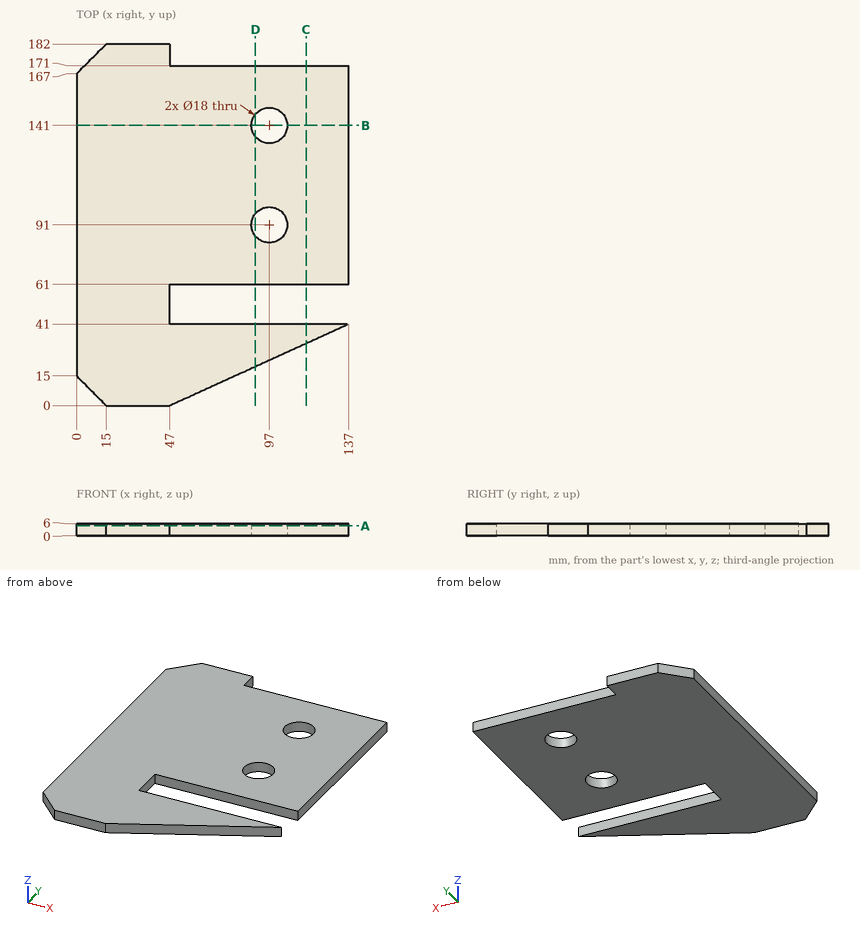
The figure shows three views and two pictorial views of one solid part (mm, origin at its lowest corner). Answer the questions. Round coordinates to 2 decimals unless told otherwise and drop trailing zeros. Write each loop counter-clockwise with the first axis right and the second up, starting at its lowest first coordinate (ties: lowest second). Pieces come first, ordered by that corner, then holes. Notation, with made-up numbers: (26, 64.25) - (51, 64.25) arc R11 ccw to (51, 72.25) - close; hole circle Ø5 at (17.5, 84.5). An arc over 180 degrees is marked (long way). Use one line per item in the form item = value. Start each with the question number.
Item 1: Find the intervals of material crossed by line 1 (X direction, y = 91, z = 2.55); line 2 (Y direction, x = 97, z = 4.05); line 3 (X direction, y = 57, z = 1.1), in increasing order. Write a range as [from, to].
Item 2: A cutting plane is placed at B-B (y = 141). Write down the section's boundary in (x, z), plus the area to 3 significant figures.
Item 3: Flat-ended cylindrical pins translate along their axes: pin 1 Ø3 at (y, z) = (47.5, 4) entering from +X; pin 2 Ø1.8 at (x, z) = (85, 3) entering from +Y; pin 3 Ø1.5 at (x, z) = (99.5, 1) entering from -Y (3 decimals). Find the tip coordinate at first contact, or state that the pin passes through.
Item 4: A cutting plane is placed at C-C (x = 115.5). Write down the section's boundary in (y, z).
Item 5: A cutting plane is placed at D-D (x = 90). Write down the section's boundary in (y, z), plus the area to 3 significant figures.
Item 6: A cutting plane is placed at A-A (z = 4.95). Write down the section's boundary in (x, y), plus the area to 3 significant figures.
The answers:
q1.line_1 = [0, 88], [106, 137]
q1.line_2 = [22.78, 41], [61, 82], [100, 132], [150, 171]
q1.line_3 = [0, 47]
q2.outline = (0, 0) - (88, 0) - (88, 6) - (0, 6) - close; (106, 0) - (137, 0) - (137, 6) - (106, 6) - close
q2.area = 714 mm^2
q3.pin_1 = 47
q3.pin_2 = 171
q3.pin_3 = 23.575
q4.outline = (31.21, 0) - (41, 0) - (41, 6) - (31.21, 6) - close; (61, 0) - (171, 0) - (171, 6) - (61, 6) - close
q5.outline = (19.59, 0) - (41, 0) - (41, 6) - (19.59, 6) - close; (61, 0) - (85.34, 0) - (85.34, 6) - (61, 6) - close; (96.66, 0) - (135.34, 0) - (135.34, 6) - (96.66, 6) - close; (146.66, 0) - (171, 0) - (171, 6) - (146.66, 6) - close
q5.area = 653 mm^2
q6.outline = (0, 15) - (15, 0) - (47, 0) - (137, 41) - (47, 41) - (47, 61) - (137, 61) - (137, 171) - (47, 171) - (47, 182) - (15, 182) - (0, 167) - close; hole circle Ø18 at (97, 91); hole circle Ø18 at (97, 141)
q6.area = 19,600 mm^2
